The drawing under review shows one solid part. Ordinate dimensions are in mm from its lowest x, y, z. Round coordinates to 2 decimals unless told otherwise and drop trailing zeros. Order: outer loops, then holes, each group sorted by start corner. A loop starts at its lowest first (then second) coordinate and runs counter-clockwise, first axis right, second up.
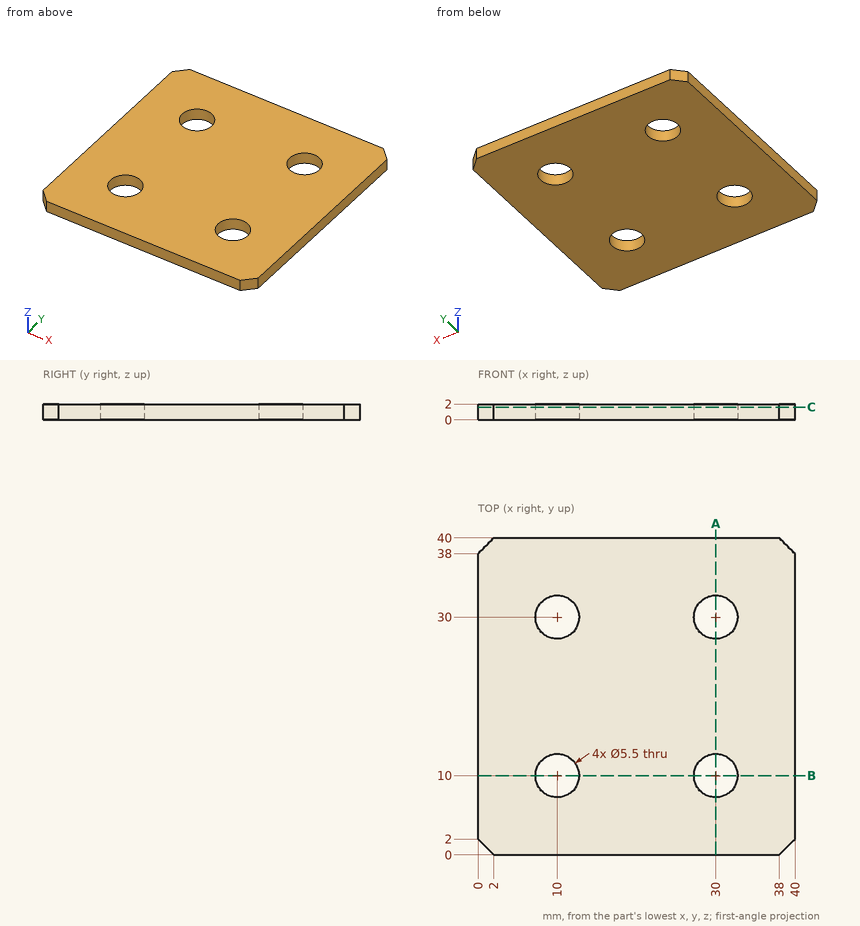
(1) To check wall thickness, follow L1, parallel to Y at x = 10, z = 0.55; L2, parallel to Y at x = 11.5, z = 0.7; L3, parallel to X at y = 10.5, z = 0.95. State the ranges of each line that lie inside material, in increasing order.
(2) We need section C-C (z = 1.6). Give the boundary of the cut face in (x, y).
(3) We need section A-A (x = 30). Give the boundary of the cut face in (y, z).
Verdict:
1. L1: y = 0 to 7.25, 12.75 to 27.25, 32.75 to 40
1. L2: y = 0 to 7.7, 12.3 to 27.7, 32.3 to 40
1. L3: x = 0 to 7.3, 12.7 to 27.3, 32.7 to 40
2. outline: (0, 2) - (2, 0) - (38, 0) - (40, 2) - (40, 38) - (38, 40) - (2, 40) - (0, 38) - close; hole circle Ø5.5 at (10, 10); hole circle Ø5.5 at (10, 30); hole circle Ø5.5 at (30, 10); hole circle Ø5.5 at (30, 30)
3. outline: (0, 0) - (7.25, 0) - (7.25, 2) - (0, 2) - close; (12.75, 0) - (27.25, 0) - (27.25, 2) - (12.75, 2) - close; (32.75, 0) - (40, 0) - (40, 2) - (32.75, 2) - close
